Geometry: see drawing. Coordinates: mm, zero at the bounding-box minimum. A direction names the side the tool comes from. Coordinates: 2 decimals unless noted, no trailing zeros. Loops run counter-clockwise (first coordinate to the right, second up) from the corner with the lowest first, then second, coordinate; pieces in that order, holes last. Notation, with made-up numbers: (59.25, -38) -> (96.25, -38) arc R23 cw to (96.25, -29) -> close; hole circle Ø8 at (-34.75, 24). An arc over 180 degrees is marked (long way). Answer as a JSON object with one key per item and string values.
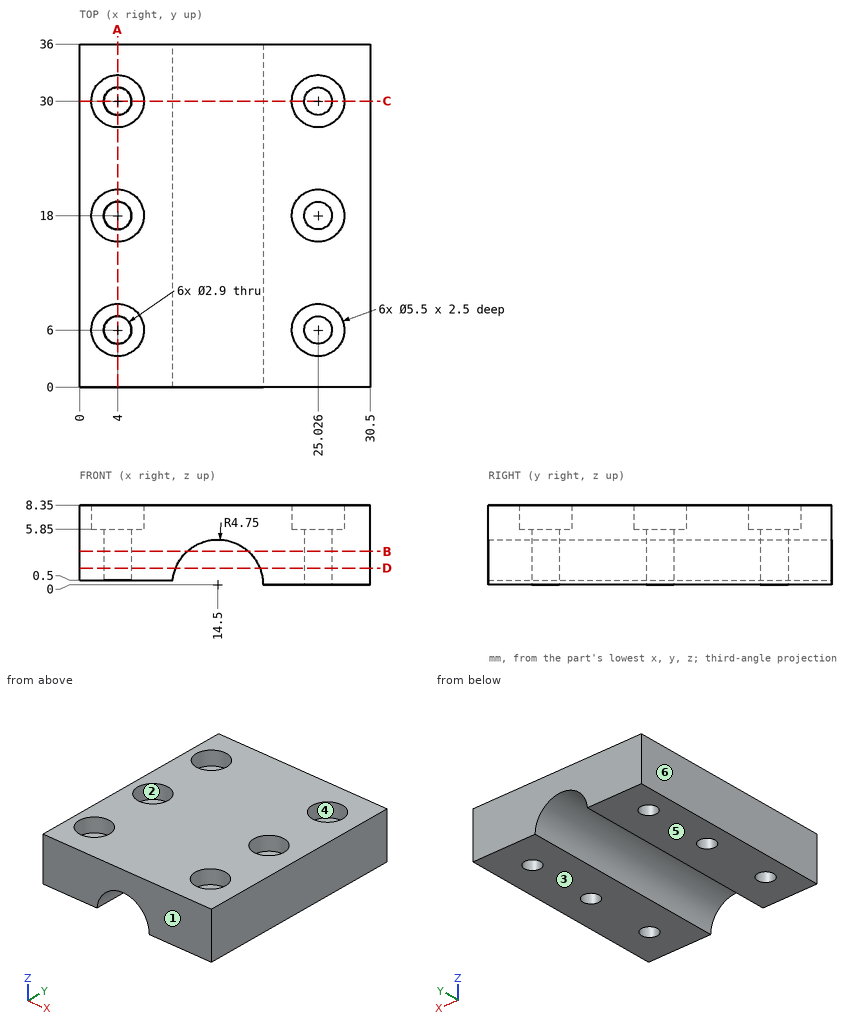
1. Line query: line 1 along Y through (x, z) = (25, 1); line 2 along Y through (x, z) = (4, 7); line 3 along X through (y, z) = (30, 6.9). Output: solid intervals per line, ascending.
Reply:
{"line 1": "y = 0 to 4.55, 7.45 to 16.55, 19.45 to 28.55, 31.45 to 36", "line 2": "y = 0 to 3.25, 8.75 to 15.25, 20.75 to 27.25, 32.75 to 36", "line 3": "x = 0 to 1.25, 6.75 to 22.28, 27.78 to 30.5"}
2. Mould query, pull axis Y, two halves, no side actions, for the marked faces 1, 2 and 3. Classes: pulls with the +Y half, pulls with the -Y half, needs draft (parallel to the pull), parting line crosses it, or undercut.
Reply:
{"face 1": "pulls with the -Y half", "face 2": "undercut", "face 3": "needs draft"}
3. Section query D-D (z = 1.75). Count the separate pieces of the cut face and the enclosed holes in it.
Reply:
{"separate pieces": "2", "enclosed holes": "6"}
4. Section query B-B (z = 3.5). Return loops of the section in (x, y), plus the area to 3 significant figures.
Reply:
{"outline": "(0, 0) -> (11.29, 0) -> (11.29, 36) -> (0, 36) -> close; (17.71, 0) -> (30.5, 0) -> (30.5, 36) -> (17.71, 36) -> close; hole circle Ø2.9 at (4, 6); hole circle Ø2.9 at (4, 18); hole circle Ø2.9 at (4, 30); hole circle Ø2.9 at (25.03, 6); hole circle Ø2.9 at (25.03, 18); hole circle Ø2.9 at (25.03, 30)", "area": "827 mm2"}
5. Pin query (flat end, axial travel): P1, Ø3, axis at x = 4, y = 19, coming from the -Z side; P2, Ø4, axis at x = 25.03, y = 30, coming from the +Z side; P3, Ø3, axis at x = 16, y = 27.5, coming from the -Z side. Return the tip coordinate at first contact, or that it passes through.
Reply:
{"P1": "stops at z = 0.5", "P2": "stops at z = 5.85", "P3": "stops at z = 3.68"}
6. Section query C-C (y = 30). Return loops of the section in (x, z), plus the area to 3 significant figures.
Reply:
{"outline": "(0, 0.5) -> (2.55, 0.5) -> (2.55, 5.85) -> (1.25, 5.85) -> (1.25, 8.35) -> (0, 8.35) -> close; (5.45, 0.5) -> (9.78, 0.5) arc R4.75 cw to (19.25, 0) -> (23.58, 0) -> (23.58, 5.85) -> (22.28, 5.85) -> (22.28, 8.35) -> (6.75, 8.35) -> (6.75, 5.85) -> (5.45, 5.85) -> close; (26.48, 0) -> (30.5, 0) -> (30.5, 8.35) -> (27.78, 8.35) -> (27.78, 5.85) -> (26.48, 5.85) -> close", "area": "154 mm2"}
7. Access query for the marked faces 4, 5 and 6. Directions: +Z, -Z, +X, -X, +Y, -Y. A direction counts if a zero-diameter tool reaches every point of the face in a straight line with its end or side. Return the directions, or none.
Reply:
{"face 4": "+Z", "face 5": "-Z, -X, +Y, -Y", "face 6": "+Z, -Z, -X, +Y, -Y"}
8. Section query A-A (x = 4). Return loops of the section in (y, z).
Reply:
{"outline": "(0, 0.5) -> (4.55, 0.5) -> (4.55, 5.85) -> (3.25, 5.85) -> (3.25, 8.35) -> (0, 8.35) -> close; (7.45, 0.5) -> (16.55, 0.5) -> (16.55, 5.85) -> (15.25, 5.85) -> (15.25, 8.35) -> (8.75, 8.35) -> (8.75, 5.85) -> (7.45, 5.85) -> close; (19.45, 0.5) -> (28.55, 0.5) -> (28.55, 5.85) -> (27.25, 5.85) -> (27.25, 8.35) -> (20.75, 8.35) -> (20.75, 5.85) -> (19.45, 5.85) -> close; (31.45, 0.5) -> (36, 0.5) -> (36, 8.35) -> (32.75, 8.35) -> (32.75, 5.85) -> (31.45, 5.85) -> close"}
